Autodesk Inventor part; units mm, degrees
ref_plane "Work Plane1" through (0, 15, 0) normal (0, 1, 0) x (-1, 0, 0)
ref_plane "YZ Plane" through (0, 0, 0) normal (1, 0, 0) x (0, 1, 0)
ref_plane "XY Plane" through (0, 0, 0) normal (0, 0, 1) x (1, 0, 0)
sketch "Sketch1" plane through (0, 0, 0) normal (0, 0, 1) x (1, 0, 0)
  line L0 (0, 0) -> (0, 20)
  line L1 (0, 0) -> (20, 0)
  arc A0 (20, 0) -> (0, 20) centre (0, 0) ccw
  line L2 (0, -4.8284) -> (0, 28.9706)
  dimension "d2" = 20
revolve "Revolution1" add sketch "Sketch1" angle 360 about axis through (0, -10, 0) along (0, 1, 0)
ref_plane "Work Plane1" through (0, 15, 0) normal (0, 1, 0) x (-1, 0, 0)
sketch "Sketch2" plane through (0, 15, 0) normal (0, 1, 0) x (-1, 0, 0)
  point P0 (0, 0)
  point P1 (0, 0)
hole "Hole1" at (0, 15, 0) direction (0, -1, 0) diameter 4.5 end through all counterbore diameter 8 counterbore depth 4
shell "Shell1" thickness 8 removed faces 1 at (13.8841, 0, 1.6858)
sketch "Sketch3" plane through (0, 0, 0) normal (0, -1, 0) x (1, 0, 0)
  circle A0 centre (0, 0) radius 10.25
  circle A1 centre (0, 0) radius 2.25
extrude "Extrusion1" cut sketch "Sketch3" against normal blind 3
properties part number "Ball_Upper Half" material "Nylon 6/6"
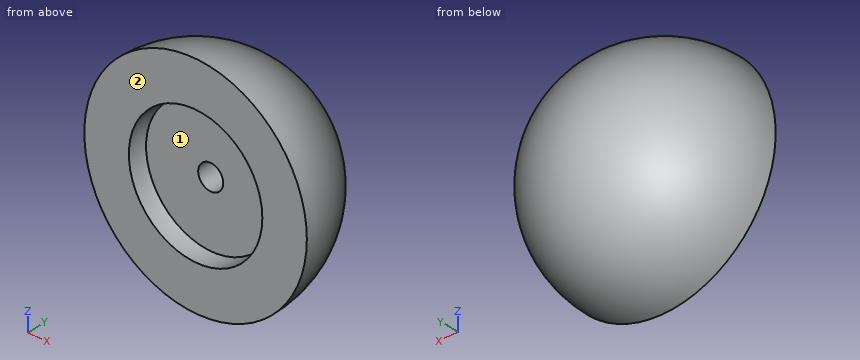
Check sheet for the modelled part. Datum: model origin and axes. Units: mm. Face numbers are marked on the shaded views. Round coordinates to 2 decimals unless told otherwise and drop trailing zeros. Order: outer loops, then holes, each group sorted by start corner. A loop starts at its lowest first (then second) coordinate and runs counter-clockwise, first axis right, second up.
1) Scan lines: line 1 (X direction, y = 5.5, z = 0); line 2 (Z direction, x = 0, y = 5.25); line 3 (Z direction, x = 0, y = 11.8). Record each from-to range of solid material in increasing order.
2) Section check A-A (z = 0). Record the boundary of the cut face in (x, y), and give its area (3 significant figures).
3) Section check D-D (x = -16). Record the boundary of the cut face in (y, z).
4) Section check B-B (x = -1). Record the boundary of the cut face in (y, z), and give its area (3 significant figures).
5) Go/stop test with flat-tipped pins: pin 1 Ø3 at (x, z) = (-2, 9.5) entering from -Y; pin 2 Ø1.5 at (x, y) = (-2.5, 17) entering from -Z; pin 3 Ø3.5 at (x, z) = (0, 0) entering from -Y. Record where each tip stops, or that it passes through.
6) Section check C-C (y = 10.25). Record the boundary of the cut face in (x, z), and give its area (3 significant figures).
7) Mould release check, pull along Z, two halves, no side actions. Record for the marked faces 1 and 2: +Z half, -Z half, draft (parallel to the pull), parting line (faces both ways), or undercut.
Result:
1. line 1: x = -19.23 to -2.25, 2.25 to 19.23
1. line 2: z = -19.3 to -2.25, 2.25 to 19.3
1. line 3: z = -16.15 to -4, 4 to 16.15
2. outline: (-20, 0) - (-12, 0) arc R12 cw to (-11.62, 3) - (-2.25, 3) - (-2.25, 11) - (-4, 11) - (-4, 15) - (4, 15) - (4, 11) - (2.25, 11) - (2.25, 3) - (11.62, 3) arc R12 cw to (12, 0) - (20, 0) arc R20 ccw to start
2. area: 489 mm2
3. outline: (0, -12) arc R12 ccw to (0, 12) - close
4. outline: (0, -19.97) arc R19.97 ccw to (0, 19.97) - (0, 11.96) arc R11.96 cw to (3, 11.58) - (3, 2.02) - (11, 2.02) - (11, 3.87) - (15, 3.87) - (15, -3.87) - (11, -3.87) - (11, -2.02) - (3, -2.02) - (3, -11.58) arc R11.96 cw to (0, -11.96) - close
4. area: 493 mm2
5. pin 1: stops at y = 3
5. pin 2: stops at z = -11.4
5. pin 3: stops at y = 15
6. outline: circle Ø34.35 at (0, 0); hole circle Ø4.5 at (0, 0)
6. area: 911 mm2
7. face 1: undercut
7. face 2: draft
